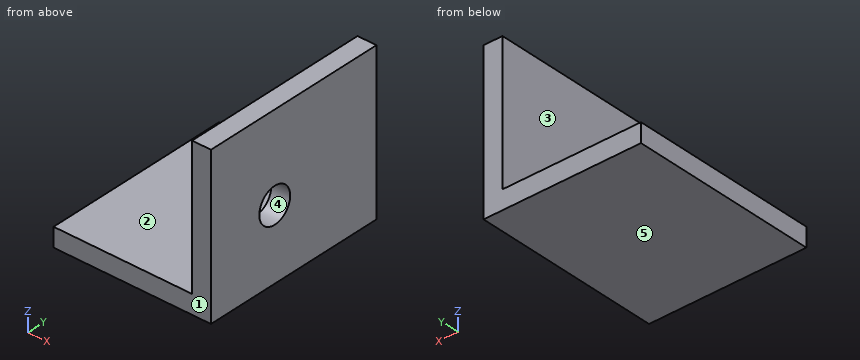
Autodesk Inventor part; units mm, degrees
ref_plane "YZ Plane" through (0, 0, 0) normal (1, 0, 0) x (0, 1, 0)
ref_plane "XZ Plane" through (0, 0, 0) normal (0, 1, 0) x (-1, 0, 0)
ref_plane "XY Plane" through (0, 0, 0) normal (0, 0, 1) x (1, 0, 0)
sketch "Sketch1" plane through (0, 0, 0) normal (0, 1, 0) x (-1, 0, 0)
  line L0 (0, 0) -> (-25, 0)
  line L1 (-25, 0) -> (-25, 3)
  line L2 (-25, 3) -> (0, 3)
  line L3 (0, 3) -> (0, 0)
  line L4 (-25, 0) -> (-22, 0)
  line L5 (-22, 0) -> (-22, 25)
  line L6 (-22, 25) -> (-25, 25)
  line L7 (-25, 25) -> (-25, 0)
  point P0 (0, 1.5)
  point P1 (-22, 3)
  dimension "d0" = 3
  dimension "d1" = 25
  dimension "d2" = 3
  dimension "d3" = 25
extrude "Extrusion1" add sketch "Sketch1" along normal blind 30
sketch "Sketch2" plane through (22, 0, 3) normal (-1, 0, 0) x (0, 0, 1)
  circle A0 centre (8.25, 11.5611) radius 2.8
  circle A1 centre (17, 32.0611) radius 1.5
  circle A2 centre (-0.5, 32.0611) radius 1.5
  point P0 (-3, 0)
extrude "Extrusion2" cut sketch "Sketch2" against normal blind 30
properties part number "connector"
CAD build for the part. Positions are in the model's coordinates, mm. Face numbers are marked on the shaded views. A direction names the side the tool comes from. Coordinates: 2 decimals unless noted, no trailing zeros. Order: outer loops, then holes, each group sorted by start corner. A loop starts at its lowest first (then second) coordinate and runs counter-clockwise, first axis right, second up. Notation, with made-up numbers: M 82,83 L 96,83 A24 ccw 96,116 Z; hole C 65,19.5 d9. An arc over 180 degrees is marked long. Write each question's results on one line, items separated by ' | '. Start each with the question number.
Q1. Cut at A-A (z = 11.25). List the corners of the cut face in (x, y), then the cut area to 3 significant figures.
Q2. Pull direction Z, two halves, no side cores. Call the marked faces 3, 4 and 5: +Z half, -Z half, draft (parallel to the pull), parting line (faces both ways), or undercut.
Q3. Drill centre lines: probe 1 along Y at (x, z) = (24, 11.25); probe 2 along Z at (x, y) = (15.75, 3.5); probe 3 along X at (y, z) = (27.5, 22.5). Where is each one in solid material? Low to high. Write a range as from..to.
Q4. Cut at C-C (x = 4). List the corners of the cut face in (y, z), then the cut area to 3 significant figures.
Q5. Cut at B-B (y = 18.5). List the corners of the cut face in (x, z), then the cut area to 3 significant figures.
Q6. Which spindle directions (+Z, -Z, +X, -X, +Y, -Y) get a long thin tool onto all of the face, cutting with end or side? Do the marked faces 1 and 2. Say none if no direction does.
Q7. Cut at D-D (z = 18.25). List the corners of the cut face in (x, y).
Q8. Flat gauge pins, fed straight in: P1, Ø5, axis at y = 11.56, z = 11.25, coming from the -X side; P2, Ø2, axis at x = 8.5, y = 23.5, coming from the -Z side; P3, Ø3, axis at x = 18, y = 7, coming from the +Z side. Where does each tip first touch, or does it go through?
Found:
1) outline: M 22,0 L 25,0 L 25,8.76 L 22,8.76 Z; M 22,14.36 L 25,14.36 L 25,30 L 22,30 Z | area: 73.2 mm²
2) face 3: draft | face 4: undercut | face 5: -Z half
3) probe 1: 0..8.76, 14.36..30 | probe 2: 0..3 | probe 3: 22..25
4) outline: M 0,0 L 30,0 L 30,3 L 0,3 Z | area: 90.0 mm²
5) outline: M 0,0 L 25,0 L 25,25 L 22,25 L 22,3 L 0,3 Z | area: 141 mm²
6) face 1: +Z, -Z, +X, -X, -Y | face 2: +Z, -X, +Y, -Y
7) outline: M 22,0 L 25,0 L 25,30 L 22,30 Z
8) P1: through | P2: z = 0 | P3: z = 3
